```python
from build123d import *

# Parameters (mm, degrees)
SKETCH1_W           = 40
SKETCH1_H           = 40
SKETCH1_R           = 7.1
BOSS_EXTRUDE1_DEPTH = 8
FILLET1_R           = 4
SKETCH2_R           = 3.15
CUT_EXTRUDE1_DEPTH  = 4.7
BOSS_EXTRUDE2_DEPTH = 8
FILLET2_R           = 4


with BuildPart() as part:
    # Sketch1 → Boss-Extrude1 (new body)
    with BuildSketch(Plane(origin=(0, 0, 0), x_dir=(1, 0, 0), z_dir=(0, 1, 0))):
        Rectangle(SKETCH1_W, SKETCH1_H)
        with Locations(Location((0, 0, 0), (0, 0, 270))):
            Circle(SKETCH1_R, mode=Mode.SUBTRACT)
        with BuildLine():
            ThreePointArc((-1.641666667, 9.712230977), (6.965001795, 6.965001795), (9.712230977, -1.641666667))
            ThreePointArc((9.712230977, -1.641666667), (11.473826233, -4.119928589), (13.952088155, -2.358333333))
            ThreePointArc((13.952088155, -2.358333333), (10.005560954, 10.005560954), (-2.358333333, 13.952088155))
            ThreePointArc((-2.358333333, 13.952088155), (-4.119928589, 11.473826233), (-1.641666667, 9.712230977))
        make_face(mode=Mode.SUBTRACT)
        with BuildLine():
            ThreePointArc((-13.952088155, 2.358333333), (-10.005560954, -10.005560954), (2.358333333, -13.952088155))
            ThreePointArc((2.358333333, -13.952088155), (4.119928589, -11.473826233), (1.641666667, -9.712230977))
            ThreePointArc((1.641666667, -9.712230977), (-6.965001795, -6.965001795), (-9.712230977, 1.641666667))
            ThreePointArc((-9.712230977, 1.641666667), (-11.473826233, 4.119928589), (-13.952088155, 2.358333333))
        make_face(mode=Mode.SUBTRACT)
    extrude(amount=BOSS_EXTRUDE1_DEPTH)

    # Fillet1
    fillet1_edges = [part.edges().sort_by_distance(p)[0] for p in [
        (-20, 4, -20),
        (20, 4, -20),
    ]]
    fillet(fillet1_edges, radius=FILLET1_R)

    # Sketch2 → Cut-Extrude1 (cut)
    with BuildSketch(Plane.XY.offset(20)):
        with Locations((-16, 4)):
            Circle(SKETCH2_R)
        with Locations((16, 4)):
            Circle(SKETCH2_R)
    extrude(amount=-CUT_EXTRUDE1_DEPTH, mode=Mode.SUBTRACT)

    # Sketch3 → Boss-Extrude2 (add)
    with BuildSketch(Plane(origin=(0, 8, 0), x_dir=(1, 0, 0), z_dir=(0, 1, 0))):
        Polygon((0, 20), (9.266942717, 36.050815617), (24.295969979, 40.077831335), (26.272725847, 37.501672932), (11.243698585, 33.474657214), (3.464101615, 20), align=None)
    extrude(amount=-BOSS_EXTRUDE2_DEPTH)

    # Fillet2
    fillet2_edges = [part.edges().sort_by_distance(p)[0] for p in [
        (3.464101615, 4, -20),
        (0, 4, -20),
    ]]
    fillet(fillet2_edges, radius=FILLET2_R)


solid = part.part
```
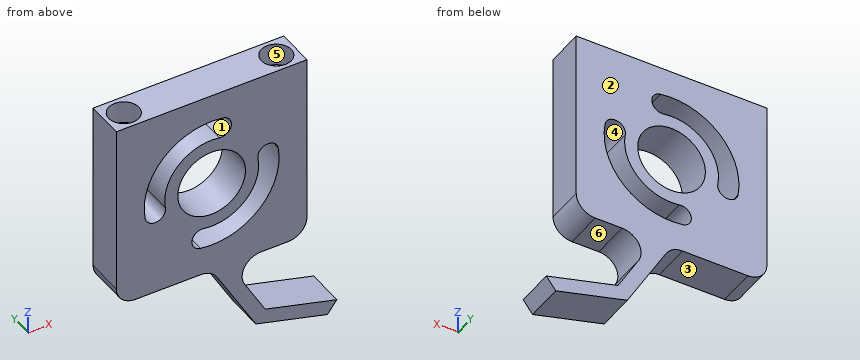
Model file for the job. Use its own axes, mm. Face numbers are marked on the shaded views. A direction names the side the tool comes from. Give positions to 0.01 mm unless a question says otherwise; leave off trailing zeros. Write each loop counter-clockwise with the first axis right and the second up, starting at its lowest first coordinate (ties: lowest second). Pieces come first, ordered by that corner, then holes. Notation, with made-up numbers: (-34, 54.5) - (25, 54.5) arc R32 cw to (25, 90.5) - close; hole circle Ø4 at (55, 23). An arc over 180 degrees is marked (long way). One line per question, with ' | ' between items. Start each with the question number.
(1) Slice it at C-C on z = -3.5. Write the cut outline in (x, y).
(2) Pin check, flat tips, straight feed: P1, Ø4, axis at x = 21.5, y = 4, coming from the -Z side; P2, Ø3, axis at x = -17.5, y = 4, coming from the +Z side; P3, Ø1, axis at y = 1, z = 10.5, coming from the +X side; P4, Ø3, axis at x = 6.5, z = -17, coming from the -Y side. Stop position of each tip, or through.
(3) Slice it at B-B on y = 2. Give the number of separate pieces and of enclosed holes in the cut face, plus the area to 3 significant figures.
(4) Slice it at D-D on x = 22.5. Write the cut outline in (y, z).
(5) 3-axis set-ups, long thin cutter, end or side, ignore diameter. For the marked faces 4, 5 and 6: which of +Z, -Z, +X, -X, +Y, -Y reach the whole face in a straight line?
(6) Two-plate mould, pull along Z, no slides. Class the marked faces 1, 2 and 3: +Z half, -Z half, draft (parallel to the pull), parting line (faces both ways), or undercut.
(7) Wall check: line 1 along X through (y, z) = (2.25, 0); line 2 along X through (y, z) = (2, -6.5); line 3 along Y through (x, z) = (16, 17). Give the ranges that are in metal, low to high. Write a range as from..to.
(8) Slice it at A-A on x = 0. Write the cut outline in (y, z).
Results below:
1) outline: (-20, 0) - (-13.37, 0) - (-13.37, 8) - (-20, 8) - close; (-10.29, 0) - (-6.18, 0) - (-6.18, 8) - (-10.29, 8) - close; (6.18, 0) - (9.21, 0) - (9.21, 8) - (6.18, 8) - close; (13.71, 0) - (20, 0) - (20, 8) - (13.71, 8) - close
2) P1: z = -39.86 | P2: z = 15.3 | P3: x = 20 | P4: y = 0
3) separate pieces: 1 | enclosed holes: 3 | area: 1,270 mm^2
4) outline: (0, -39.6) - (8, -39.6) - (8, -36.49) - (0, -36.49) - close
5) face 4: +Y, -Y | face 5: +Z | face 6: +X, +Y, -Y
6) face 1: undercut | face 2: draft | face 3: -Z half
7) line 1: -20..-14.15, -9.85..-7.1, 7.1..9.85, 14.15..20 | line 2: -20..-2.86, 2.86..7.4, 12.57..20 | line 3: 0..0.85, 7.15..8
8) outline: (0, -20.73) - (8, -20.73) - (8, -14.15) - (0, -14.15) - close; (0, -9.85) - (8, -9.85) - (8, -7.1) - (0, -7.1) - close; (0, 7.1) - (8, 7.1) - (8, 9.85) - (0, 9.85) - close; (0, 14.15) - (8, 14.15) - (8, 20) - (0, 20) - close
